from build123d import *

# Parameters (mm, degrees)
CROQUIS1_W              = 45
CROQUIS1_H              = 7.5
CROQUIS1_R              = 1.6
SALIENTE_EXTRUIR1_DEPTH = 7.5
CORTAR_EXTRUIR1_REACH   = 9.5
CROQUIS2_R              = 1.6
CORTAR_EXTRUIR2_DEPTH   = 3
CORTAR_EXTRUIR3_DEPTH   = 3


with BuildPart() as part:
    # Croquis1 → Saliente-Extruir1 (new body)
    with BuildSketch(Plane.XY):
        Rectangle(CROQUIS1_W, CROQUIS1_H)
        with Locations((-17.5, 0)):
            Circle(CROQUIS1_R, mode=Mode.SUBTRACT)
        with Locations((17.5, 0)):
            Circle(CROQUIS1_R, mode=Mode.SUBTRACT)
    extrude(amount=SALIENTE_EXTRUIR1_DEPTH)

    # Croquis2 → Cortar-Extruir1 (cut, up to next)
    with BuildSketch(Plane(origin=(0, 3.75, 0), x_dir=(1, 0, 0), z_dir=(0, 1, 0)), mode=Mode.PRIVATE) as cortar_extruir1_sk1:
        with Locations((0, -3.75)):
            Circle(CROQUIS2_R)
    cortar_extruir1_tool1 = extrude(cortar_extruir1_sk1.sketch, amount=-CORTAR_EXTRUIR1_REACH, mode=Mode.PRIVATE) & part.part
    add(cortar_extruir1_tool1.solids().sort_by_distance((0, 3.75, 3.75))[0], mode=Mode.SUBTRACT)

    # Croquis3 → Cortar-Extruir2 (cut)
    with BuildSketch(Plane.XZ.offset(3.75)):
        Polygon((3.290896534, 3.75), (1.645448267, 6.6), (-1.645448267, 6.6), (-3.290896534, 3.75), (-1.645448267, 0.9), (1.645448267, 0.9), align=None)
    extrude(amount=-CORTAR_EXTRUIR2_DEPTH, mode=Mode.SUBTRACT)

    # Croquis4 → Cortar-Extruir3 (cut)
    with BuildSketch(Plane.XY.offset(7.5)):
        Polygon((-14.209103466, 0), (-15.854551733, 2.85), (-19.145448267, 2.85), (-20.790896534, 0), (-19.145448267, -2.85), (-15.854551733, -2.85), align=None)
        Polygon((20.790896534, 0), (19.145448267, 2.85), (15.854551733, 2.85), (14.209103466, 0), (15.854551733, -2.85), (19.145448267, -2.85), align=None)
    extrude(amount=-CORTAR_EXTRUIR3_DEPTH, mode=Mode.SUBTRACT)


solid = part.part
Geometry: final body of the model. Coordinates: model frame, mm. A direction names the side the tool comes from. Coordinates: 2 decimals unless noted, no trailing zeros. Order: outer loops, then holes, each group sorted by start corner. A loop starts at its lowest first (then second) coordinate and runs counter-clockwise, first axis right, second up. Notation, with made-up numbers: (-29, 79) - (29, 79) arc R18 ccw to (29, 97) - close; hole circle Ø4 at (28.25, -1.75). An arc over 180 degrees is marked (long way). Use one line per item in the form item = value.
1) Set-up query: faces 4 (the face through (19.96, -1.44, 6.02)), 5 (the face through (-0.3, -3.75, 0.4)), 6 (the face through (2.46, -2.27, 2.31)). Return all of +Z, -Z, +X, -X, +Y, -Y with unobstructed straight access to the full face (end or side cutting, diameter ignored); none if empty.
Solutions:
face_4 = +Z
face_5 = +Z, -Z, +X, -X, -Y
face_6 = -Y
2) Section D-D (x = 18.5). Return loops of the section in (y, z).
Solutions:
outline = (-3.75, 0) - (-1.25, 0) - (-1.25, 4.5) - (-2.85, 4.5) - (-2.85, 7.5) - (-3.75, 7.5) - close; (1.25, 0) - (3.75, 0) - (3.75, 7.5) - (2.85, 7.5) - (2.85, 4.5) - (1.25, 4.5) - close
3) Mould query, pull axis Z, two halves, no side actions, for faces 1 (the face through (-2.46, -2.27, 5.19)), 2 (the face through (0, 0, 7.5)), 3 (the face through (-15.02, 1.405, 6.021)). Classes: +Z half, -Z half, draft (parallel to the pull), parting line (faces both ways), or undercut.
Solutions:
face_1 = undercut
face_2 = +Z half
face_3 = draft
4) Ray query, L1, parallel to X at y = 0, z = 0.9; L2, parallel to Y at x = 17.5, z = 1.8; L3, parallel to Z at x = 0, y = 1.8. Return the intervals inside material, ascending.
Solutions:
L1 = -22.5 to -19.1, -15.9 to 15.9, 19.1 to 22.5
L2 = -3.75 to -1.6, 1.6 to 3.75
L3 = 0 to 2.15, 5.35 to 7.5
5) Section C-C (z = 0.5). Return loops of the section in (x, y).
Solutions:
outline = (-22.5, -3.75) - (22.5, -3.75) - (22.5, 3.75) - (-22.5, 3.75) - close; hole circle Ø3.2 at (-17.5, 0); hole circle Ø3.2 at (17.5, 0)
6) Section B-B (z = 3.25). Return loops of the section in (x, y).
Solutions:
outline = (-22.5, -3.75) - (-3, -3.75) - (-3, -0.75) - (-1.52, -0.75) - (-1.52, 3.75) - (-22.5, 3.75) - close; (1.52, -0.75) - (3, -0.75) - (3, -3.75) - (22.5, -3.75) - (22.5, 3.75) - (1.52, 3.75) - close; hole circle Ø3.2 at (-17.5, 0); hole circle Ø3.2 at (17.5, 0)
7) Pin query (flat end, axial travel): pin 1 (3 mm diameter, centred on x = -16, y = -1, fed in from +Z). Return the tip coordinate at first contact, or that it passes through.
Solutions:
pin_1 = 7.5
8) Section A-A (x = -17.5). Return loops of the section in (y, z).
Solutions:
outline = (-3.75, 0) - (-1.6, 0) - (-1.6, 4.5) - (-2.85, 4.5) - (-2.85, 7.5) - (-3.75, 7.5) - close; (1.6, 0) - (3.75, 0) - (3.75, 7.5) - (2.85, 7.5) - (2.85, 4.5) - (1.6, 4.5) - close
